Here's the drawing with two shaded views (mm, measured from the low corner). I have some questions. A direction names the side the tool comes from. Round coordinates to 2 decimals unless told otherwise and drop trailing zeros. Order: outer loops, then holes, each group sorted by start corner. A loop starts at its lowest first (then second) coordinate and runs counter-clockwise, first axis right, second up. Notation, with made-up numbers: (15.5, -38) - (38.5, -38) arc R20 cw to (38.5, -3) - close; hole circle Ø11 at (66, 78.5). An arc over 180 degrees is marked (long way). One line per item, written item: value.
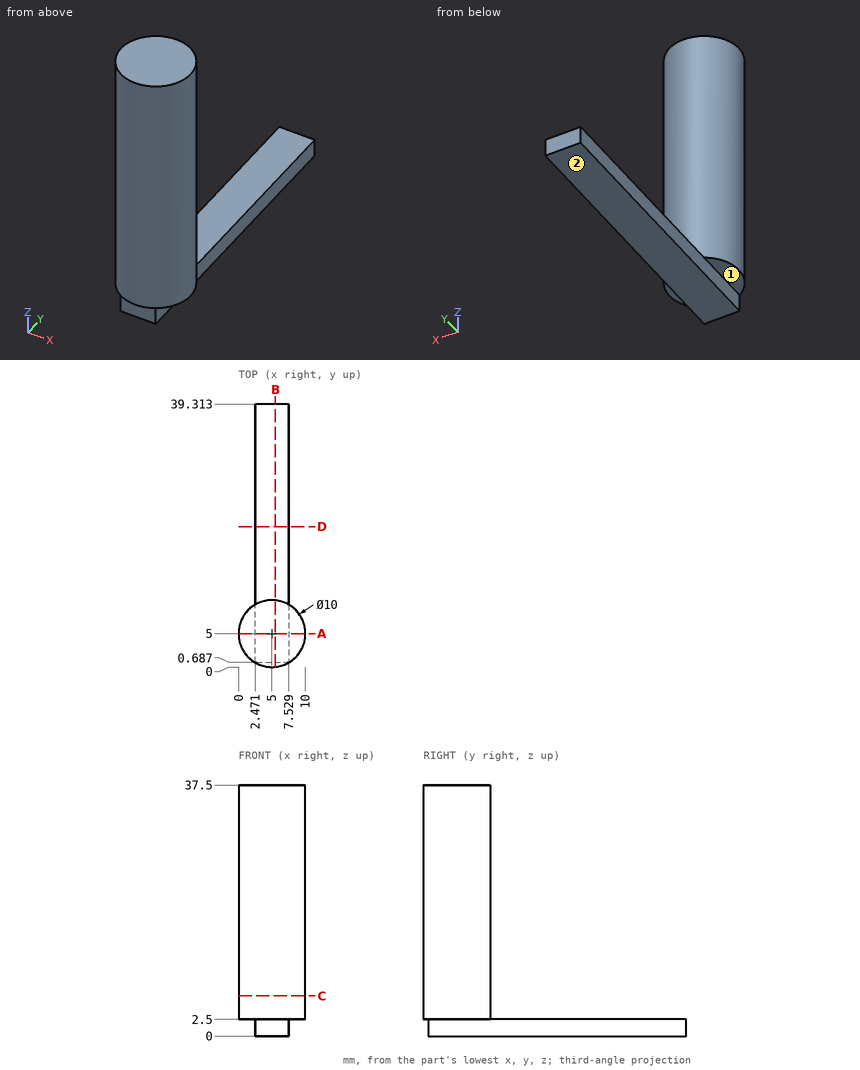
Q1. Which directions (+Z, -Z, +X, -X, +Y, -Y) give clear straight access to the entire face, cutting with the end or side of a thin tool? Please do the marked faces 1 and 2.
Results list:
face 1: -Z, -X, +Y, -Y
face 2: -Z, +X, -X, +Y, -Y
Q2. If we section it at D-D, the plane y = 21: Please give me the cut outline in (x, z).
Results list:
outline: (2.47, 0) - (7.53, 0) - (7.53, 2.5) - (2.47, 2.5) - close
Q3. If we section it at B-B, the plane x = 5.5: Please give me the cut outline in (y, z) (1 decimal).
Results list:
outline: (0, 2.5) - (0.7, 2.5) - (0.7, 0) - (39.3, 0) - (39.3, 2.5) - (10, 2.5) - (10, 37.5) - (0, 37.5) - close
Q4. If I drill on line 1 along Z through (x, y) = (3.75, 31.5); line 2 along Y through (x, z) = (7, 21); line 3 along Y through (x, z) = (8.25, 9.5), over which ranges is the centre line in solid material (lowest first)?
Results list:
line 1: 0 to 2.5
line 2: 0.42 to 9.58
line 3: 1.2 to 8.8
Q5. If we section it at A-A, the plane y = 5: Please give me the cut outline in (x, z), then the cut area to 3 significant figures.
Results list:
outline: (0, 2.5) - (2.47, 2.5) - (2.47, 0) - (7.53, 0) - (7.53, 2.5) - (10, 2.5) - (10, 37.5) - (0, 37.5) - close
area: 363 mm²
Q6. Will these pins go through, and if not, where does the flat tip stop? pin 1 (3 mm diameter, centred on x = 5.5, z = 26.5, fed in from +Y); pin 2 (0.8 mm diameter, centred on x = 6, y = 0.5, fed in from -Z); pin 3 (1.2 mm diameter, centred on y = 28.5, z = 1.5, fed in from +X); pin 4 (1.2 mm diameter, centred on x = 4, z = 1.5, fed in from -Y).
Results list:
pin 1: y = 10
pin 2: z = 0
pin 3: x = 7.53
pin 4: y = 0.69
Q7. If we section it at C-C, the plane z = 6: Please give me the cut outline in (x, y).
Results list:
outline: circle Ø10 at (5, 5)
